Design review of the part built by this model. Coordinates are the model's own, in mm. A direction names the side the tool comes from. Round coordinates to 2 decimals unless told otherwise and drop trailing zeros. Loops run counter-clockwise (first coordinate to the right, second up) from the corner with the lowest first, then second, coordinate; pieces in that order, holes last. Notation, with made-up numbers: M 12,22.25 L 50,22.25 A14 ccw 50,44.25 Z; hole C -10,66 d3. An arc over 180 degrees is marked long. Use a Markdown table: item, result.
from build123d import *

# Parameters (mm, degrees)
SKETCH_1_R          = 23
EXTRUDE_1_DEPTH     = 25
SKETCH_2_R          = 1.5
SKETCH_2_R_2        = 2.6
CUT_EXTRUDE_1_DEPTH = 10
SKETCH_3_R          = 2.6
EXTRUDE_2_DEPTH     = 27
CHAMFER_1_SIZE      = 10
CUT_EXTRUDE_2_DEPTH = 9.5
SKETCH_5_R          = 1.595744681
CUT_EXTRUDE_3_DEPTH = 2
SKETCH_6_R          = 2.6
CUT_EXTRUDE_4_DEPTH = 12
SKETCH_7_R          = 2
EXTRUDE_3_DEPTH     = 5
EXTRUDE_4_DEPTH     = 5
CUT_EXTRUDE_5_DEPTH = 5
SKETCH_10_R         = 1.595744681
EXTRUDE_5_DEPTH     = 2.4
CUT_EXTRUDE_6_DEPTH = 1.4
SKETCH_12_R         = 1.2
CUT_EXTRUDE_7_DEPTH = 5


with BuildPart() as part:
    # 草图1 → 凸台-拉伸1 (new body)
    with BuildSketch(Plane.XY):
        Circle(SKETCH_1_R)
    extrude(amount=EXTRUDE_1_DEPTH)

    # 草图2 → 切除-拉伸1 (cut)
    with BuildSketch(Plane(origin=(0, 0, 0), x_dir=(-1, 0, 0), z_dir=(0, 0, -1))):
        with Locations((6, 0)):
            Circle(SKETCH_2_R)
        with Locations((0, -6)):
            Circle(SKETCH_2_R)
        with Locations((-6, 0)):
            Circle(SKETCH_2_R)
        with Locations((0, 6)):
            Circle(SKETCH_2_R)
        Circle(SKETCH_2_R_2)
    extrude(amount=-CUT_EXTRUDE_1_DEPTH, mode=Mode.SUBTRACT)

    # 草图3 → 凸台-拉伸2 (add)
    with BuildSketch(Plane(origin=(0, 0, 10), x_dir=(-1, 0, 0), z_dir=(0, 0, -1))):
        Circle(SKETCH_3_R)
    extrude(amount=-EXTRUDE_2_DEPTH)

    # 倒角1
    chamfer_1_edges = [part.edges().sort_by_distance(p)[0] for p in [
        (-23, 0, 0),
    ]]
    chamfer(chamfer_1_edges, length=CHAMFER_1_SIZE)

    # 草图4 → 切除-拉伸2 (cut)
    with BuildSketch(Plane(origin=(0, 0, 0), x_dir=(-1, 0, 0), z_dir=(0, 0, -1))):
        with BuildLine():
            ThreePointArc((3.800832161, -12.431961828), (3.264127324, -12.583539757), (2.72141518, -12.711958913))
            Line((2.72141518, -12.711958913), (8.204578209, -21.486854037))
            ThreePointArc((8.204578209, -21.486854037), (16.263455967, -16.263455967), (21.486854037, -8.204578209))
            Line((21.486854037, -8.204578209), (12.711958913, -2.72141518))
            ThreePointArc((12.711958913, -2.72141518), (9.578191182, -8.789667439), (3.800832161, -12.431961828))
        make_face()
        with BuildLine():
            ThreePointArc((12.711958913, -2.72141518), (6.363961031, -6.363961031), (2.72141518, -12.711958913))
            ThreePointArc((2.72141518, -12.711958913), (3.264127324, -12.583539757), (3.800832161, -12.431961828))
            ThreePointArc((3.800832161, -12.431961828), (9.578191182, -8.789667439), (12.711958913, -2.72141518))
        make_face()
        with BuildLine():
            ThreePointArc((2.72141518, 12.711958913), (6.363961031, 6.363961031), (12.711958913, 2.72141518))
            ThreePointArc((12.711958913, 2.72141518), (9.192388155, 9.192388155), (2.72141518, 12.711958913))
        make_face()
        with BuildLine():
            ThreePointArc((2.72141518, 12.711958913), (9.192388155, 9.192388155), (12.711958913, 2.72141518))
            Line((12.711958913, 2.72141518), (21.486854037, 8.204578209))
            ThreePointArc((21.486854037, 8.204578209), (16.263455967, 16.263455967), (8.204578209, 21.486854037))
            Line((8.204578209, 21.486854037), (2.72141518, 12.711958913))
        make_face()
        with BuildLine():
            Line((-21.486854037, 8.204578209), (-12.711958913, 2.72141518))
            ThreePointArc((-12.711958913, 2.72141518), (-9.192388155, 9.192388155), (-2.72141518, 12.711958913))
            Line((-2.72141518, 12.711958913), (-8.204578209, 21.486854037))
            ThreePointArc((-8.204578209, 21.486854037), (-16.263455967, 16.263455967), (-21.486854037, 8.204578209))
        make_face()
        with BuildLine():
            ThreePointArc((-2.72141518, 12.711958913), (-9.192388155, 9.192388155), (-12.711958913, 2.72141518))
            ThreePointArc((-12.711958913, 2.72141518), (-6.363961031, 6.363961031), (-2.72141518, 12.711958913))
        make_face()
        with BuildLine():
            Line((-8.204578209, -21.486854037), (-2.72141518, -12.711958913))
            ThreePointArc((-2.72141518, -12.711958913), (-9.192388155, -9.192388155), (-12.711958913, -2.72141518))
            Line((-12.711958913, -2.72141518), (-21.486854037, -8.204578209))
            ThreePointArc((-21.486854037, -8.204578209), (-16.263455967, -16.263455967), (-8.204578209, -21.486854037))
        make_face()
        with BuildLine():
            ThreePointArc((-12.711958913, -2.72141518), (-9.192388155, -9.192388155), (-2.72141518, -12.711958913))
            ThreePointArc((-2.72141518, -12.711958913), (-6.363961031, -6.363961031), (-12.711958913, -2.72141518))
        make_face()
    extrude(amount=-CUT_EXTRUDE_2_DEPTH, mode=Mode.SUBTRACT)

    # 草图5 → 切除-拉伸3 (cut)
    with BuildSketch(Plane.XY.offset(25)):
        with Locations((0, 12.5)):
            Circle(SKETCH_5_R)
        with Locations((12.5, 0)):
            Circle(SKETCH_5_R)
        with Locations((0, -12.5)):
            Circle(SKETCH_5_R)
        with Locations((-12.5, 0)):
            Circle(SKETCH_5_R)
    extrude(amount=-CUT_EXTRUDE_3_DEPTH, mode=Mode.SUBTRACT)

    # 草图6 → 切除-拉伸4 (cut)
    with BuildSketch(Plane.XY.offset(37)):
        Circle(SKETCH_6_R)
    extrude(amount=-CUT_EXTRUDE_4_DEPTH, mode=Mode.SUBTRACT)

    # 草图7 → 凸台-拉伸3 (add)
    with BuildSketch(Plane.XY.offset(25)):
        Circle(SKETCH_7_R)
    extrude(amount=EXTRUDE_3_DEPTH)

    # 草图8 → 凸台-拉伸4 (add)
    with BuildSketch(Plane.XY.offset(25)):
        Polygon((17.67766953, -24.748737342), (24.748737342, -17.67766953), (17.597575781, -10.526507969), (10.526507969, -17.597575781), align=None)
    extrude(amount=-EXTRUDE_4_DEPTH)

    # 草图9 → 切除-拉伸5 (cut)
    with BuildSketch(Plane.XY.offset(25)):
        with BuildLine():
            Line((-17.335793171, 14.790208759), (-17.486366766, 14.940782353))
            ThreePointArc((-17.486366766, 14.940782353), (-18.615341136, 13.50811143), (-19.627234895, 11.990481658))
            Line((-19.627234895, 11.990481658), (-15.839191899, 8.202438662))
            Line((-15.839191899, 8.202438662), (-13.293607486, 10.748023074))
            Line((-13.293607486, 10.748023074), (-17.335793171, 14.790208759))
        make_face()
        with BuildLine():
            Line((-8.202438662, 15.839191899), (-11.990481658, 19.627234895))
            ThreePointArc((-11.990481658, 19.627234895), (-13.50811143, 18.615341136), (-14.940782353, 17.486366766))
            Line((-14.940782353, 17.486366766), (-14.790208759, 17.335793171))
            Line((-14.790208759, 17.335793171), (-10.748023074, 13.293607486))
            Line((-10.748023074, 13.293607486), (-8.202438662, 15.839191899))
        make_face()
        with BuildLine():
            Line((8.202438662, 15.839191899), (10.748023074, 13.293607486))
            Line((10.748023074, 13.293607486), (14.790208759, 17.335793171))
            Line((14.790208759, 17.335793171), (14.940782353, 17.486366766))
            ThreePointArc((14.940782353, 17.486366766), (13.50811143, 18.615341136), (11.990481658, 19.627234895))
            Line((11.990481658, 19.627234895), (8.202438662, 15.839191899))
        make_face()
        with BuildLine():
            ThreePointArc((19.627234895, 11.990481658), (18.615341136, 13.50811143), (17.486366766, 14.940782353))
            Line((17.486366766, 14.940782353), (17.335793171, 14.790208759))
            Line((17.335793171, 14.790208759), (13.293607486, 10.748023074))
            Line((13.293607486, 10.748023074), (15.839191899, 8.202438662))
            Line((15.839191899, 8.202438662), (19.627234895, 11.990481658))
        make_face()
        with BuildLine():
            Line((-14.790208759, -17.335793171), (-14.940782353, -17.486366766))
            ThreePointArc((-14.940782353, -17.486366766), (-13.50811143, -18.615341136), (-11.990481658, -19.627234895))
            Line((-11.990481658, -19.627234895), (-8.202438662, -15.839191899))
            Line((-8.202438662, -15.839191899), (-10.748023074, -13.293607486))
            Line((-10.748023074, -13.293607486), (-14.790208759, -17.335793171))
        make_face()
        with BuildLine():
            Line((-15.839191899, -8.202438662), (-19.627234895, -11.990481658))
            ThreePointArc((-19.627234895, -11.990481658), (-18.615341136, -13.50811143), (-17.486366766, -14.940782353))
            Line((-17.486366766, -14.940782353), (-17.335793171, -14.790208759))
            Line((-17.335793171, -14.790208759), (-13.293607486, -10.748023074))
            Line((-13.293607486, -10.748023074), (-15.839191899, -8.202438662))
        make_face()
    extrude(amount=-CUT_EXTRUDE_5_DEPTH, mode=Mode.SUBTRACT)

    # 草图10 → 凸台-拉伸5 (add)
    with BuildSketch(Plane.XY.offset(25)):
        with BuildLine():
            Line((-10.748023074, -13.293607486), (-8.202438662, -15.839191899))
            Line((-8.202438662, -15.839191899), (-11.990481658, -19.627234895))
            ThreePointArc((-11.990481658, -19.627234895), (0.205316668, -22.99908357), (12.33897396, -19.410041772))
            Line((12.33897396, -19.410041772), (17.67766953, -24.748737342))
            Line((17.67766953, -24.748737342), (24.748737342, -17.67766953))
            Line((24.748737342, -17.67766953), (19.410041772, -12.33897396))
            ThreePointArc((19.410041772, -12.33897396), (22.99908357, -0.205316668), (19.627234895, 11.990481658))
            Line((19.627234895, 11.990481658), (15.839191899, 8.202438662))
            Line((15.839191899, 8.202438662), (13.293607486, 10.748023074))
            Line((13.293607486, 10.748023074), (17.486366766, 14.940782353))
            ThreePointArc((17.486366766, 14.940782353), (16.263455967, 16.263455967), (14.940782353, 17.486366766))
            Line((14.940782353, 17.486366766), (10.748023074, 13.293607486))
            Line((10.748023074, 13.293607486), (8.202438662, 15.839191899))
            Line((8.202438662, 15.839191899), (11.990481658, 19.627234895))
            ThreePointArc((11.990481658, 19.627234895), (0, 23), (-11.990481658, 19.627234895))
            Line((-11.990481658, 19.627234895), (-8.202438662, 15.839191899))
            Line((-8.202438662, 15.839191899), (-10.748023074, 13.293607486))
            Line((-10.748023074, 13.293607486), (-14.940782353, 17.486366766))
            ThreePointArc((-14.940782353, 17.486366766), (-16.263455967, 16.263455967), (-17.486366766, 14.940782353))
            Line((-17.486366766, 14.940782353), (-13.293607486, 10.748023074))
            Line((-13.293607486, 10.748023074), (-15.839191899, 8.202438662))
            Line((-15.839191899, 8.202438662), (-19.627234895, 11.990481658))
            ThreePointArc((-19.627234895, 11.990481658), (-23, 0), (-19.627234895, -11.990481658))
            Line((-19.627234895, -11.990481658), (-15.839191899, -8.202438662))
            Line((-15.839191899, -8.202438662), (-13.293607486, -10.748023074))
            Line((-13.293607486, -10.748023074), (-17.486366766, -14.940782353))
            ThreePointArc((-17.486366766, -14.940782353), (-16.263455967, -16.263455967), (-14.940782353, -17.486366766))
            Line((-14.940782353, -17.486366766), (-10.748023074, -13.293607486))
        make_face()
        with Locations((0, 12.5)):
            Circle(SKETCH_10_R, mode=Mode.SUBTRACT)
        with Locations((-12.5, 0)):
            Circle(SKETCH_10_R, mode=Mode.SUBTRACT)
        with Locations((0, -12.5)):
            Circle(SKETCH_10_R, mode=Mode.SUBTRACT)
        with Locations((12.5, 0)):
            Circle(SKETCH_10_R, mode=Mode.SUBTRACT)
    extrude(amount=EXTRUDE_5_DEPTH)

    # 草图11 → 切除-拉伸6 (cut)
    with BuildSketch(Plane(origin=(0, 0, 20), x_dir=(-1, 0, 0), z_dir=(0, 0, -1))):
        with BuildLine():
            Line((-17.67766953, -24.748737342), (-12.33897396, -19.410041772))
            ThreePointArc((-12.33897396, -19.410041772), (-16.263455967, -16.263455967), (-19.410041772, -12.33897396))
            Line((-19.410041772, -12.33897396), (-24.748737342, -17.67766953))
            Line((-24.748737342, -17.67766953), (-17.67766953, -24.748737342))
        make_face()
    extrude(amount=-CUT_EXTRUDE_6_DEPTH, mode=Mode.SUBTRACT)

    # 草图12 → 切除-拉伸7 (cut)
    with BuildSketch(Plane.XY.offset(27.4)):
        with Locations((15.454813221, 4.141104722)):
            Circle(SKETCH_12_R)
        with Locations((-4.141104722, -15.454813221)):
            Circle(SKETCH_12_R)
        with Locations((-11.313708499, 11.313708499)):
            Circle(SKETCH_12_R)
    extrude(amount=-CUT_EXTRUDE_7_DEPTH, mode=Mode.SUBTRACT)


solid = part.part
1. Wall thickness on line 1 along X through (y, z) = (14.5, 22.25); line 2 along Z through (x, y) = (3, 2); line 3 along Z through (x, y) = (12.5, -13): over which ranges is each line inside the solid? List them lowest first. Write a range as from..to.
Check values:
| item | result |
|---|---|
| line 1 | x = -17.05..-11.95, -9.54..9.54, 11.95..17.05 |
| line 2 | z = 0..27.4 |
| line 3 | z = 9.5..27.4 |
2. The part is to be moulded in two halves that separate along X. For faces 1 (the face through (22.12, -15.05, 24.36)), 2 (the face through (1.52, -12.02, 25.17)), 3 (the face through (3, 0, 0)), 4 (the face through (12, 0, 23)), say which applies: pulls with the +X half, pulls with the -X half, needs draft (parallel to the pull), parting line crosses it, or undercut.
Check values:
| item | result |
|---|---|
| face 1 | pulls with the +X half |
| face 2 | undercut |
| face 3 | needs draft |
| face 4 | undercut |
3. Machinability: for faces 5 (the face through (0.325, -7.464, 4.93)), 6 (the face through (-14.55, 9.49, 23.65)), 7 (the face through (4.712, 15.898, 5.739)), which of the approach directions +Z, -Z, +X, -X, +Y, -Y give a long, thin tool a straight path to every point of the face, cutting with its end or side? Answer none if there is none.
Check values:
| item | result |
|---|---|
| face 5 | -Z |
| face 6 | +Z |
| face 7 | -Z, +X |
4. Take a section at B-B on z = 26. Count the separate pieces of the cut face and the enclosed holes in it, and give its area (3 significant figures).
Check values:
| item | result |
|---|---|
| separate pieces | 1 |
| enclosed holes | 7 |
| area | 1,570 mm² |
5. Take a section at C-C on z = 16.75. Give the boundary of the cut face in (x, y).
Check values:
| item | result |
|---|---|
| outline | C 0,0 d46 |
6. Insertion check: pin 1 (2.5 mm diameter, centred on x = 12, y = -0.5, fed in from +Z); pin 2 (3 mm diameter, centred on x = -14.5, y = -10, fed in from -Z); pin 3 (10 mm diameter, centred on x = 14.5, z = 7, fed in from +Y); pin 4 (12 mm diameter, centred on x = -14, y = -4, fed in from -Z). Each pin has a flat end and moves straight along its axis. Give the tip position at first contact, or say it passes through.
Check values:
| item | result |
|---|---|
| pin 1 | stops at z = 27.4 |
| pin 2 | stops at z = 9.5 |
| pin 3 | stops at y = 20.46 |
| pin 4 | stops at z = 0 |
